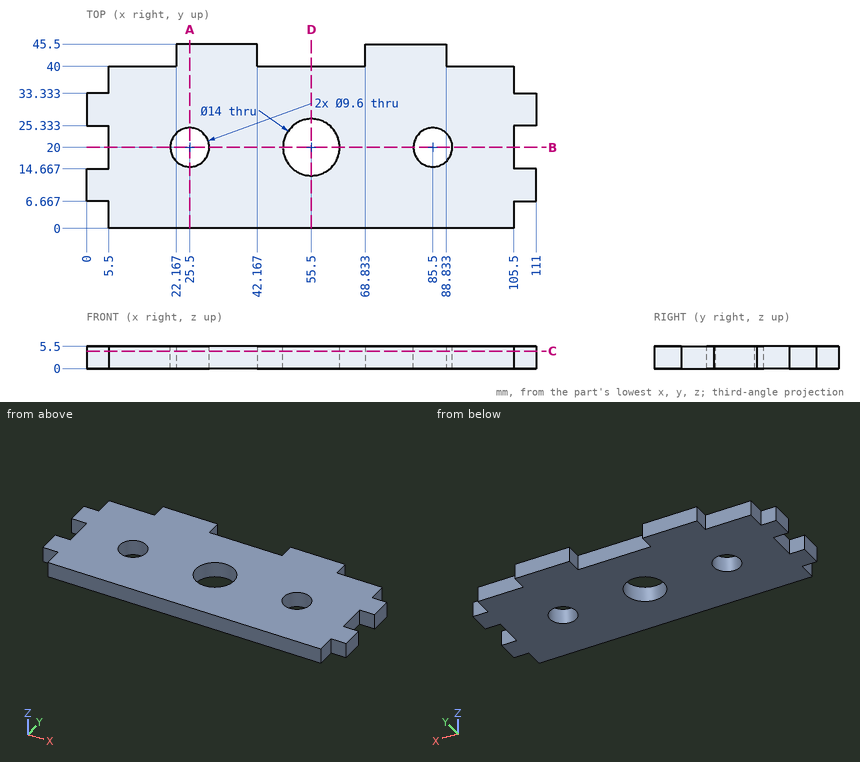
Design review of the part shown in the three views and the two pictorial views. Dimensions are in mm from the part's minimum x, y and z. Coordinates: 2 decimals unless noted, no trailing zeros. Order: outer loops, then holes, each group sorted by start corner. A loop starts at its lowest first (then second) coordinate and runs counter-clockwise, first axis right, second up.
Item 1: Take a section at B-B, the plane y = 20. Write out the cut boundary in (x, z).
Item 2: For line 1 (X direction, y = 20, z = 3.35); line 2 (Y direction, x = 106.5, z = 1.1); line 3 (X direction, y = 42, z = 0.2), list the stretches that pass through material, from the lowest coordinate up.
Item 3: Take a section at C-C, the plane z = 4.3. Count the separate pieces of the cut face and the enclosed holes in it, then the cut area to 3 significant figures.
Item 4: Take a section at D-D, the plane x = 55.5. Write out the cut boundary in (y, z).
Item 5: For pin 1 Ø3 at (y, z) = (42.5, 3.5) entering from -X; pin 2 Ø8.5 at (x, y) = (85.5, 20) entering from +Z; pin 3 Ø3 at (y, z) = (2.5, 1.5) entering from -X; pin 4 Ø1.6 at (x, z) = (109.5, 2.5) entering from +Y, all flat-tipped, find the tip position at first contact; note any pin that passes through.
Item 6: Take a section at A-A, the plane x = 25.5. Write out the cut boundary in (y, z).
The answers:
1. outline: (5.5, 0) - (20.7, 0) - (20.7, 5.5) - (5.5, 5.5) - close; (30.3, 0) - (48.5, 0) - (48.5, 5.5) - (30.3, 5.5) - close; (62.5, 0) - (80.7, 0) - (80.7, 5.5) - (62.5, 5.5) - close; (90.3, 0) - (105.5, 0) - (105.5, 5.5) - (90.3, 5.5) - close
2. line 1: x = 5.5 to 20.7, 30.3 to 48.5, 62.5 to 80.7, 90.3 to 105.5
2. line 2: y = 6.67 to 14.67, 25.33 to 33.33
2. line 3: x = 22.17 to 42.17, 68.83 to 88.83
3. separate pieces: 1
3. enclosed holes: 3
3. area: 4,100 mm2
4. outline: (0, 0) - (13, 0) - (13, 5.5) - (0, 5.5) - close; (27, 0) - (40, 0) - (40, 5.5) - (27, 5.5) - close
5. pin 1: stops at x = 22.17
5. pin 2: passes through
5. pin 3: stops at x = 5.5
5. pin 4: stops at y = 33.33
6. outline: (0, 0) - (15.2, 0) - (15.2, 5.5) - (0, 5.5) - close; (24.8, 0) - (45.5, 0) - (45.5, 5.5) - (24.8, 5.5) - close
